Geometry: final body of the model. Coordinates: model frame, mm. A direction names the side the tool comes from. Give positions to 0.01 mm unless a question says otherwise; leave off trailing zeros. Write each loop counter-clockwise with the first axis right and the second up, starting at its lowest first coordinate (ties: lowest second). Pieces come first, ordered by that corner, then holes. Notation, with made-up numbers: (64.25, -33.5) - (82.25, -33.5) arc R20 ccw to (82.25, -10.5) - close; hole circle Ø9 at (75, 59.25). An arc over 180 degrees is marked (long way). Return JSON: item names as keys, results as strings.
from build123d import *

# Parameters (mm, degrees)
SKETCH1_W           = 492.125
SKETCH1_H           = 274.6375
BOSS_EXTRUDE1_DEPTH = 4.7625
CUT_EXTRUDE1_REACH  = 6.763


with BuildPart() as part:
    # Sketch1 → Boss-Extrude1 (new body)
    with BuildSketch(Plane(origin=(0, 0, 0), x_dir=(0, 0, -1), z_dir=(1, 0, 0))):
        Rectangle(SKETCH1_W, SKETCH1_H)
    extrude(amount=BOSS_EXTRUDE1_DEPTH)

    # Sketch2 → Cut-Extrude1 (cut, up to next)
    with BuildSketch(Plane(origin=(4.7625, 0, 0), x_dir=(0, 0, -1), z_dir=(1, 0, 0)), mode=Mode.PRIVATE) as cut_extrude1_sk1:
        Polygon((-24.852813742, -60), (24.852813742, -60), (42.426406871, -42.426406871), (60, -24.852813742), (60, 24.852813742), (24.852813742, 60), (-24.852813742, 60), (-60, 24.852813742), (-60, -24.852813742), align=None)
    cut_extrude1_tool1 = extrude(cut_extrude1_sk1.sketch, amount=-CUT_EXTRUDE1_REACH, mode=Mode.PRIVATE) & part.part
    add(cut_extrude1_tool1.solids().sort_by_distance((4.7625, 0, 0))[0], mode=Mode.SUBTRACT)


solid = part.part
Q1. Mould query, pull axis Y, two halves, no side actions, for faces 3 (the flat face through (0, 63, 3)), 4 (the flat face through (2.41, -42.18, 42.67)). Classes: pulls with the +Y half, pulls with the -Y half, needs draft (parallel to the pull), parting line crosses it, or undercut.
Answer key:
{"face 3": "needs draft", "face 4": "undercut"}
Q2. Set-up query: faces 1 (the flat face through (2.41, 42.18, -42.67)), 2 (the flat face through (4.762, 63, 3)). Return all of +Z, -Z, +X, -X, +Y, -Y with unobstructed straight access to the full face (end or side cutting, diameter ignored); none if empty.
Answer key:
{"face 1": "+X, -X", "face 2": "+Z, -Z, +X, +Y, -Y"}
Q3. Section query B-B, the plane x = 1.85. Return the cut outline in (y, z).
Answer key:
{"outline": "(-137.32, -246.06) - (137.32, -246.06) - (137.32, 246.06) - (-137.32, 246.06) - close; hole (-60, -24.85) - (-24.85, -60) - (24.85, -60) - (60, -24.85) - (60, 24.85) - (24.85, 60) - (-24.85, 60) - (-60, 24.85) - close"}
Q4. Material intervals for probe 1 along Y at (x, z) = (4.5, 56.5); probe 2 along Z at (x, y) = (1.35, 25); probe 3 along Z at (x, y) = (3.9, 26), sorted ascending. Write a range as [from, to].
Answer key:
{"probe 1": "y = [-137.32, -28.35], [28.35, 137.32]", "probe 2": "z = [-246.06, -59.85], [59.85, 246.06]", "probe 3": "z = [-246.06, -58.85], [58.85, 246.06]"}
Q5. Section query A-A, the plane z = 11.5. Return the cut outline in (x, y).
Answer key:
{"outline": "(0, -137.32) - (4.76, -137.32) - (4.76, -60) - (0, -60) - close; (0, 60) - (4.76, 60) - (4.76, 137.32) - (0, 137.32) - close"}
Q6. Section query C-C, the plane y = -41. Return the cut outline in (x, z), plus the area to 3 significant figures.
Answer key:
{"outline": "(0, -246.06) - (4.76, -246.06) - (4.76, -43.85) - (0, -43.85) - close; (0, 43.85) - (4.76, 43.85) - (4.76, 246.06) - (0, 246.06) - close", "area": "1,930 mm^2"}
